Here's how the part is built. I have some questions about the finished solid (model axes, mm). Face numbers are marked on the shaded views. Coordinates: 2 decimals unless noted, no trailing zeros. Order: outer loops, then holes, each group sorted by start corner. A loop starts at its lowest first (then second) coordinate and runs counter-clockwise, first axis right, second up. Notation, with made-up numbers: (39.5, -24.75) -> (61.5, -24.75) arc R8 ccw to (61.5, -15.75) -> close; hole circle Ø11 at (-9.5, 24). An arc over 180 degrees is marked (long way). One line per item, written item: value. Start each with the question number.
Autodesk Fusion 360 part; units mm, degrees
sketch "Sketch1" plane through (0, 0, 0) normal (0, 0, 1) x (1, 0, 0)
  line L0 (-96.825, 55.325) -> (96.825, 55.325)
  line L1 (96.825, 55.325) -> (96.825, -55.325)
  line L2 (96.825, -55.325) -> (-96.825, -55.325)
  line L3 (-96.825, -55.325) -> (-96.825, 55.325)
  line L4 (-86.825, 52.575) -> (86.825, 52.575)
  line L5 (86.825, 52.575) -> (86.825, -52.575)
  line L6 (86.825, -52.575) -> (-86.825, -52.575)
  line L7 (-86.825, -52.575) -> (-86.825, 52.575)
  point P0 (0, 55.325)
  point P1 (96.825, 0)
  point P2 (0, 52.575)
  point P3 (86.825, 0)
  dimension "d1" = 193.65
  dimension "d2" = 110.65
  dimension "d9" = 2.75
  dimension "d10" = 10
extrude "Extrude2" add sketch "Sketch1" along normal mid plane 8
fillet "Fillet1" radius 7.5 4 edges at (-96.825, 55.325, 0) (-96.825, -55.325, 0) (96.825, -55.325, 0) (96.825, 55.325, 0)
sketch "Sketch2" plane through (0, 0, 4) normal (0, 0, 1) x (-1, 0, 0)
  arc A0 (-96.825, -47.825) -> (-89.325, -55.325) centre (-89.325, -47.825) ccw
  line L0 (-89.325, -55.325) -> (89.325, -55.325)
  arc A1 (89.325, -55.325) -> (96.825, -47.825) centre (89.325, -47.825) ccw
  line L1 (96.825, -47.825) -> (96.825, 47.825)
  arc A2 (96.825, 47.825) -> (89.325, 55.325) centre (89.325, 47.825) ccw
  line L2 (89.325, 55.325) -> (-89.325, 55.325)
  arc A3 (-89.325, 55.325) -> (-96.825, 47.825) centre (-89.325, 47.825) ccw
  line L3 (-96.825, 47.825) -> (-96.825, -47.825)
  line L4 (-86.825, 52.575) -> (86.825, 52.575)
  line L5 (86.825, 52.575) -> (86.825, -52.575)
  line L6 (86.825, -52.575) -> (-86.825, -52.575)
  line L7 (-86.825, -52.575) -> (-86.825, 52.575)
  line L8 (96.825, -47.825) -> (96.825, 47.825)
  arc A4 (96.825, 47.825) -> (89.325, 55.325) centre (89.325, 47.825) ccw
  line L9 (89.325, 55.325) -> (-89.325, 55.325)
  arc A5 (-89.325, 55.325) -> (-96.825, 47.825) centre (-89.325, 47.825) ccw
  line L10 (-96.825, 47.825) -> (-96.825, -47.825)
  arc A6 (-96.825, -47.825) -> (-89.325, -55.325) centre (-89.325, -47.825) ccw
  line L11 (-89.325, -55.325) -> (89.325, -55.325)
  arc A7 (89.325, -55.325) -> (96.825, -47.825) centre (89.325, -47.825) ccw
extrude "Extrude3" add sketch "Sketch2" along normal blind 6 contours A0 L0 A1 L1 A2 L2 A3 L3 L8 A4 L9 A5 L10 A6 L11 A7 | L4 L5 L6 L7
sketch "Sketch3" plane through (0, 0, 10) normal (0, 0, 1) x (-1, 0, 0)
  arc A0 (89.325, -55.325) -> (96.825, -47.825) centre (89.325, -47.825) ccw
  line L0 (96.825, -47.825) -> (96.825, 47.825)
  arc A1 (96.825, 47.825) -> (89.325, 55.325) centre (89.325, 47.825) ccw
  line L1 (89.325, 55.325) -> (-89.325, 55.325)
  arc A2 (-89.325, 55.325) -> (-96.825, 47.825) centre (-89.325, 47.825) ccw
  line L2 (-96.825, 47.825) -> (-96.825, -47.825)
  arc A3 (-96.825, -47.825) -> (-89.325, -55.325) centre (-89.325, -47.825) ccw
  line L3 (-89.325, -55.325) -> (89.325, -55.325)
  line L4 (72.305, -37.575) -> (-68.825, -37.575) construction
  line L5 (-68.825, -37.575) -> (-68.825, 35.975) construction
  line L6 (-68.825, 35.975) -> (72.305, 35.975) construction
  line L7 (72.305, 35.975) -> (72.305, -37.575) construction
  point P0 (-61.325, -33.575)
  point P1 (-61.325, 31.975)
  point P2 (64.805, -33.575)
  point P3 (64.805, 31.975)
  dimension "d17" = 73.55
  dimension "d18" = 4
  dimension "d19" = 4
  dimension "d20" = 141.13
  dimension "d21" = 7.5
  dimension "d22" = 7.5
  dimension "d23" = 4
  dimension "d24" = 7.5
  dimension "d25" = 4
  dimension "d26" = 7.5
  dimension "d27" = 28
  dimension "d28" = 17.75
extrude "Extrude5" cut 1 faces at (28.9417, -17.525, 4) along direction (0, 0, 1) blind 2
sketch "Sketch4" plane through (0, 0, 10) normal (0, 0, 1) x (-1, 0, 0)
  arc A0 (89.325, -55.325) -> (96.825, -47.825) centre (89.325, -47.825) ccw
  line L0 (96.825, -47.825) -> (96.825, 47.825)
  arc A1 (96.825, 47.825) -> (89.325, 55.325) centre (89.325, 47.825) ccw
  line L1 (89.325, 55.325) -> (-89.325, 55.325)
  arc A2 (-89.325, 55.325) -> (-96.825, 47.825) centre (-89.325, 47.825) ccw
  line L2 (-96.825, 47.825) -> (-96.825, -47.825)
  arc A3 (-96.825, -47.825) -> (-89.325, -55.325) centre (-89.325, -47.825) ccw
  line L3 (-89.325, -55.325) -> (89.325, -55.325)
  line L4 (55, -45) -> (-55, -45)
  line L5 (-55, -45) -> (-55, 45)
  line L6 (-55, 45) -> (55, 45)
  line L7 (55, 45) -> (55, -45)
  point P0 (0, -45)
  dimension "d33" = 110
  dimension "d35" = 45
  dimension "d36" = 45
extrude "Extrude4" cut sketch "Sketch4" against normal through all contours L4 L5 L6 L7
sketch "Sketch5" plane through (0, 0, 6) normal (0, 0, -1) x (1, 0, 0)
  line L0 (86.825, -52.575) -> (86.825, 52.575)
  line L1 (86.825, 52.575) -> (-86.825, 52.575)
  line L2 (-86.825, 52.575) -> (-86.825, -52.575)
  line L3 (-86.825, -52.575) -> (86.825, -52.575)
  circle A0 centre (61.325, -33.575) radius 7.5
  circle A1 centre (61.325, 31.975) radius 7.5
  circle A2 centre (-64.805, -33.575) radius 7.5
  circle A3 centre (-64.805, 31.975) radius 7.5
  line L4 (-55, -45) -> (-55, 45)
  line L5 (-55, 45) -> (55, 45)
  line L6 (55, 45) -> (55, -45)
  line L7 (55, -45) -> (-55, -45)
  line L8 (-64.805, -26.075) -> (-55, -26.075)
  line L9 (-64.805, -41.075) -> (-55, -41.075)
  line L10 (-64.805, 39.475) -> (-55, 39.475)
  line L11 (-64.805, 24.475) -> (-55, 24.475)
  line L12 (61.325, 39.475) -> (55, 39.475)
  line L13 (61.325, 24.475) -> (55, 24.475)
  line L14 (61.325, -26.075) -> (55, -26.075)
  line L15 (61.325, -41.075) -> (55, -41.075)
  point P0 (61.325, -33.575)
  point P1 (-64.805, -33.575)
  point P2 (-64.805, 31.975)
  point P3 (61.325, 31.975)
  dimension "d39" = 15
  dimension "d47" = 126.13
extrude "Extrude6" add sketch "Sketch5" along normal blind 2 contours A0 L6 | A0 L6 L14 | A0 L6 L15 | A1 L6 L13 | A1 L6 | A1 L6 L12 | A2 L4 L8 L9 | A2 | A3 L4 L10 L11 | A3 picked at (59.7964, -33.5066) picked at (59.5829, 32.3308)
sketch "Sketch6" plane through (0, 0, 10) normal (0, 0, 1) x (-1, 0, 0)
  line L0 (55, 45) -> (55, -45)
  line L1 (55, -45) -> (-55, -45)
  line L2 (-55, -45) -> (-55, 45)
  line L3 (-55, 45) -> (55, 45)
  arc A0 (89.325, -55.325) -> (96.825, -47.825) centre (89.325, -47.825) ccw
  line L4 (96.825, -47.825) -> (96.825, 47.825)
  arc A1 (96.825, 47.825) -> (89.325, 55.325) centre (89.325, 47.825) ccw
  line L5 (89.325, 55.325) -> (-89.325, 55.325)
  arc A2 (-89.325, 55.325) -> (-96.825, 47.825) centre (-89.325, 47.825) ccw
  line L6 (-96.825, 47.825) -> (-96.825, -47.825)
  arc A3 (-96.825, -47.825) -> (-89.325, -55.325) centre (-89.325, -47.825) ccw
  line L7 (-89.325, -55.325) -> (89.325, -55.325)
  circle A4 centre (64.805, -33.575) radius 5
  circle A5 centre (64.805, 31.975) radius 5
  circle A6 centre (-61.325, -33.575) radius 5
  circle A7 centre (-61.325, 31.975) radius 5
  line L8 (64.805, -38.575) -> (55, -38.575)
  line L9 (64.805, -28.575) -> (55, -28.575)
  line L10 (64.805, 26.975) -> (55, 26.975)
  line L11 (64.805, 36.975) -> (55, 36.975)
  line L12 (-61.325, 36.975) -> (-55, 36.975)
  line L13 (-61.325, 26.975) -> (-55, 26.975)
  line L14 (-61.325, -28.575) -> (-55, -28.575)
  line L15 (-61.325, -38.575) -> (-55, -38.575)
  point P0 (64.805, -33.575)
  point P1 (64.805, 31.975)
  point P2 (-61.325, 31.975)
  point P3 (-61.325, -33.575)
  dimension "d44" = 10
extrude "Extrude7" cut sketch "Sketch6" against normal blind 4 contours L0 A5 L10 L11 | A5 | L2 A7 L12 L13 | L0 A4 L8 L9 | A7 | A4 | L2 A6 L14 L15 | A6
hole "Hole1" at (-64.805, 33.575, 10) at (61.325, 33.575, 10) at (61.325, -31.975, 10) at (-64.805, -31.975, 10) direction (0, 0, -1) diameter 3.4 end through all counterbore diameter 6.5 counterbore depth 3
fillet "Fillet3" radius 1 8 edges at (-55, 28.575, 8) (-55, 38.575, 8) (55, 38.575, 8) (55, 28.575, 8) (55, -26.975, 8) (55, -36.975, 8) (-55, -26.975, 8) (-55, -36.975, 8)
fillet "Fillet4" radius 2 12 edges at (-59.9025, -24.475, 6) (-72.305, -31.975, 6) (-59.9025, -39.475, 6) (-59.9025, 41.075, 6) (-72.305, 33.575, 6) (-59.9025, 26.075, 6) (58.1625, 26.075, 6) (68.825, 33.575, 6) (58.1625, 41.075, 6) (58.1625, -39.475, 6) (68.825, -31.975, 6) (58.1625, -24.475, 6)
equation "d1 = 193.75 mm - 0.1 mm"
equation "d2 = 110.75 mm - 0.1 mm"
equation "d9 = 2.00 mm + 0.75 mm"
equation "d11 = 6 mm + 2 mm"
equation "d19 = d18"
equation "d22 = d21"
equation "d23 = d18"
equation "d24 = d21"
equation "d25 = d23"
equation "d26 = d24"
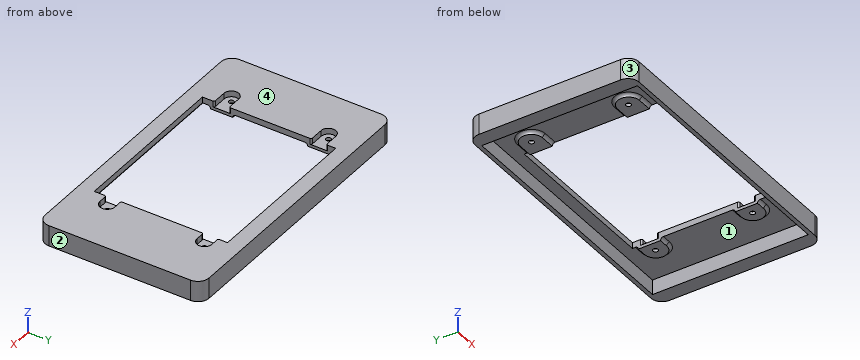
Q1. I need wall thicknesses on line 1 (Y direction, x = -3.5, z = -3) (3 decimals); line 2 (Y direction, x = 48, z = 7.75) (3 decimals); line 3 (X direction, y = -9, z = 0) (3 decimals). Which ranges of each line are inside material? Lowest first, please.
Q2. Imagine slicing it at C-C (z = -1.75). Write out the boundary of the cut face in (x, y) (3 decimals), plus the area to 3 significant figures.
Q3. Imagine slicing it at B-B (x = -14). Write out the boundary of the cut face in (y, z) (3 decimals), plus the area to 3 significant figures.
Q4. For P1, Ø10, axis at x = -73.5, y = 43, coming from the -Z side, with a flat end and sliding along its axis, tell me the tip position at first contact or that it passes through.
Q5. Imagine slicing it at A-A (y = 15). Write out the boundary of the cut face in (x, z) (3 decimals), plus the area to 3 significant figures.
Q6. If we mould it in two halves opening along X, with no side actions, what happens to the marked faces 1, 2, 3 and 4? For each: +X half, -X half, draft (parallel to the pull), parting line (faces both ways), or undercut.
Completed:
1. line 1: y = -55.325 to -52.575, 52.575 to 55.325
1. line 2: y = -55.325 to -45, 45 to 55.325
1. line 3: x = -96.825 to -86.825, 86.825 to 96.825
2. outline: (-96.825, -47.825) arc R7.5 ccw to (-89.325, -55.325) -> (89.325, -55.325) arc R7.5 ccw to (96.825, -47.825) -> (96.825, 47.825) arc R7.5 ccw to (89.325, 55.325) -> (-89.325, 55.325) arc R7.5 ccw to (-96.825, 47.825) -> close; hole (-86.825, -52.575) -> (86.825, -52.575) -> (86.825, 52.575) -> (-86.825, 52.575) -> close
2. area: 3,120 mm2
3. outline: (-55.325, -4) -> (-52.575, -4) -> (-52.575, 6) -> (-45, 6) -> (-45, 10) -> (-55.325, 10) -> close; (45, 6) -> (52.575, 6) -> (52.575, -4) -> (55.325, -4) -> (55.325, 10) -> (45, 10) -> close
3. area: 138 mm2
4. P1: stops at z = 5.09
5. outline: (-96.825, -4) -> (-86.825, -4) -> (-86.825, 6) -> (-55, 6) -> (-55, 10) -> (-96.825, 10) -> close; (55, 6) -> (86.825, 6) -> (86.825, -4) -> (96.825, -4) -> (96.825, 10) -> (55, 10) -> close
5. area: 535 mm2
6. face 1: undercut
6. face 2: +X half
6. face 3: -X half
6. face 4: draft
